The model under review builds one solid part; all positions refer to its coordinate system, in mm. Face numbers are marked on the shaded views. Coordinates: 2 decimals unless noted, no trailing zeros. Order: outer loops, then holes, each group sorted by start corner. A loop starts at its lowest first (then second) coordinate and runs counter-clockwise, first axis right, second up.
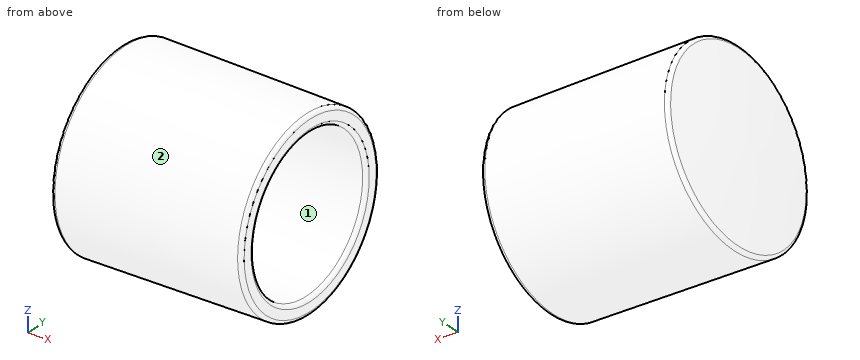
Autodesk Inventor part; units mm, degrees
ref_plane "YZ Plane" through (0, 0, 0) normal (1, 0, 0) x (0, 1, 0)
ref_plane "XZ Plane" through (0, 0, 0) normal (0, 1, 0) x (-1, 0, 0)
ref_plane "XY Plane" through (0, 0, 0) normal (0, 0, 1) x (1, 0, 0)
sketch "Sketch1" plane through (0, 0, 0) normal (0, 1, 0) x (-1, 0, 0)
  line L0 (0, 0) -> (13, 0) construction
  line L1 (0.25, 5) -> (11, 5)
  line L2 (11, 5) -> (11, 0)
  line L3 (0, 5.25) -> (0, 5.8529)
  line L4 (13, 0) -> (13, 6.25) construction
  line L5 (12.2781, 6.2417) -> (0.2471, 6.1029)
  arc A0 (13, 0) -> (12.5289, 6.0237) centre (-46.977, -1.6605) ccw
  arc A1 (0.2471, 6.1029) -> (0, 5.8529) centre (0.25, 5.8529) ccw
  arc A2 (0, 5.25) -> (0.25, 5) centre (0.25, 5.25) ccw
  arc A3 (12.5289, 6.0237) -> (12.2781, 6.2417) centre (12.281, 5.9917) ccw
  line L6 (13, 0) -> (11, 0)
  point P0 (0, 5)
  point P1 (0, 6.1)
  point P2 (12.5, 6.2442)
  dimension "d0" = 13
  dimension "d1" = 11
  dimension "d2" = 5
  dimension "d3" = 1.1
  dimension "d5" = 2
  dimension "d6" = 6.25
  dimension "d7" = 60
  dimension "d8" = 0.5
  dimension "d9" = 0.25
revolve "Revolution1" add sketch "Sketch1" angle 360 about axis through (0, 0, 0) along (-1, 0, 0)
properties part number "10mm_Endcap" material "Rubber"
(1) Consider section A-A (x = -1.5). Give the boundary of the cut face in (y, z).
(2) Wall thickness on line 1 (Y direction, x = -4.5, z = 1.75); line 2 (Z direction, x = -1.25, y = 1.5); line 3 (Y direction, x = -9.75, z = 1.5): over which ranges is each line inside the solid? List them lowest first.
(3) The part is to be moulded in two halves that separate along Y. For the marked faces 1 and 2, say which applies: +Y half, -Y half, draft (parallel to the pull), parting line (faces both ways), or undercut.
(4) Insertion check: pin 1 Ø2 at (x, y) = (-7, 1) entering from +Z; pin 2 Ø1 at (y, z) = (-0.5, -1) entering from -X; pin 3 Ø5 at (y, z) = (4, 1.5) entering from -X. Each pin has a flat end and moves straight along its axis. Give the tip position at first contact, or say it passes through.
(5) Consider section B-B (x = -3.5). Give the boundary of the cut face in (y, z).
Findings:
1. outline: circle Ø12.23 at (0, 0); hole circle Ø10 at (0, 0)
2. line 1: y = -5.9 to -4.68, 4.68 to 5.9
2. line 2: z = -5.93 to -4.77, 4.77 to 5.93
2. line 3: y = -6.03 to -4.77, 4.77 to 6.03
3. face 1: undercut
3. face 2: parting line
4. pin 1: stops at z = 6.19
4. pin 2: stops at x = -12.98
4. pin 3: stops at x = -12.92
5. outline: circle Ø12.28 at (0, 0); hole circle Ø10 at (0, 0)
